Could you check a few things on this model? Use its own coordinates, in mm. Coordinates: 2 decimals unless noted, no trailing zeros. Write each loop counter-clockwise with the first axis right and the second up, starting at its lowest first coordinate (ties: lowest second). Pieces come first, ordered by that corner, then holes.
Item 1: I want a section at A-A on x = 25.5. Please give me the cut outline in (y, z).
Item 2: If I drill on probe 1 along Y at (x, z) = (317.5, 3.1); probe 2 along Y at (x, z) = (317, 3.15); probe 3 along X at (y, z) = (27, 2.2), over which ranges is the centre line in solid material (lowest first)?
Item 3: For P1, Ø4, axis at x = 292.1, y = 12.7, coming from the -Z side, with a flat end and sliding along its axis, tell me the tip position at first contact or that it passes through.
Item 4: I want a section at B-B on z = 1.95. State how many separate pieces and enclosed holes the cut face has, then the cut area to 3 significant figures.
from build123d import *

# Parameters (mm, degrees)
SKETCH1_W                          = 330.2
SKETCH1_H                          = 50.8
BASE_DEPTH                         = 4.064
F_10_CLEARANCE_HOLE_BASKET_MOUNT_D = 5.1054
PIVOT_HOLE_DEPTH                   = 5.064
F_10_CLEARANCE_HOLE1_D             = 5.1054


with BuildPart() as part:
    # Sketch1 → base (new body)
    with BuildSketch(Plane.XY):
        with Locations((165.1, 25.4)):
            Rectangle(SKETCH1_W, SKETCH1_H)
    extrude(amount=BASE_DEPTH)

    # #10 Clearance Hole - basket mount (through all)
    with Locations(Plane.XY.offset(4.064)):
        with Locations((203.2, 12.7), (228.6, 38.1), (203.2, 38.1), (228.6, 12.7), (76.2, 38.1), (101.6, 12.7), (76.2, 12.7), (101.6, 38.1)):
            Hole(F_10_CLEARANCE_HOLE_BASKET_MOUNT_D / 2)

    # Sketch7 → pivot hole (cut, through all)
    with BuildSketch(Plane.XY.offset(4.064)):
        Polygon((21.733825791, 31.75), (18.067651581, 25.4), (21.733825791, 19.05), (29.066174209, 19.05), (32.732348419, 25.4), (29.066174209, 31.75), align=None)
    extrude(amount=-PIVOT_HOLE_DEPTH, mode=Mode.SUBTRACT)

    # #10 Clearance Hole1 (through all)
    with Locations(Plane.XY.offset(4.064)):
        with Locations((317.5, 38.1), (292.1, 12.7), (317.5, 12.7), (292.1, 38.1)):
            Hole(F_10_CLEARANCE_HOLE1_D / 2)


solid = part.part
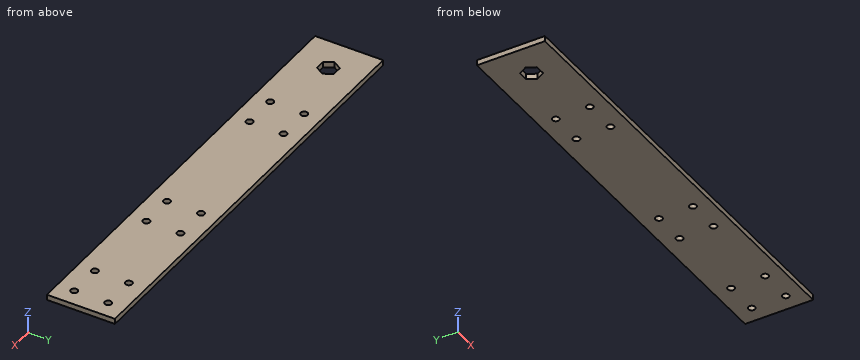
Response values:
1. outline: (0, 0) - (19.05, 0) - (19.05, 4.06) - (0, 4.06) - close; (31.75, 0) - (50.8, 0) - (50.8, 4.06) - (31.75, 4.06) - close
2. probe 1: y = 0 to 10.15, 15.25 to 35.55, 40.65 to 50.8
2. probe 2: y = 0 to 10.2, 15.2 to 35.6, 40.6 to 50.8
2. probe 3: x = 0 to 18.99, 31.81 to 330.2
3. P1: passes through
4. separate pieces: 1
4. enclosed holes: 13
4. area: 16,400 mm2
